```python
from build123d import *

# Parameters (mm, degrees)
F0_R     = 12.425
F0_R_2   = 11.175
F1_DEPTH = 38.1
F0_R_3   = 18.425
F2_DEPTH = 2.5
F3_SIZE  = 2
F4_R     = 1
F5_W     = 26.7045460641
F5_H     = 56.1363650486
F6_DEPTH = 1
F8_DEPTH = 50


with BuildPart() as f1:
    # F0 (on Top) → F1 (new body)
    with BuildSketch(Plane.XY):
        Circle(F0_R)
        Circle(F0_R_2, mode=Mode.SUBTRACT)
    extrude(amount=-F1_DEPTH)

    # F0 (on Top) → F2 (join)
    with BuildSketch(Plane.XY):
        Circle(F0_R_3)
        Circle(F0_R, mode=Mode.SUBTRACT)
        Circle(F0_R)
        Circle(F0_R_2, mode=Mode.SUBTRACT)
    extrude(amount=F2_DEPTH)

    # F3
    f3_edges = [f1.edges().sort_by_distance(p)[0] for p in [
        (-18.425, 0, 2.5),
    ]]
    chamfer(f3_edges, length=F3_SIZE)

    # F4
    f4_edges = [f1.edges().sort_by_distance(p)[0] for p in [
        (-11.175, 0, 2.5),
    ]]
    fillet(f4_edges, radius=F4_R)

    # F5 (on Right) → F6 (cut)
    with BuildSketch(Plane.YZ):
        with Locations((13.3522730321, -17.5000005402)):
            Rectangle(F5_W, F5_H)
    extrude(amount=-F6_DEPTH, mode=Mode.SUBTRACT)

    # F7 (on Top) → F8 (cut, symmetric)
    with BuildSketch(Plane.XY):
        Polygon((5.7434663265, -25.6659543005), (0, -11.8), (-5.7434663265, -25.6659543005), align=None)
    extrude(amount=F8_DEPTH, both=True, mode=Mode.SUBTRACT)


solid = f1.part
```
Here's how the part is built. I have some questions about the finished solid (model axes, mm). A direction names the side the tool comes from. Round coordinates to 2 decimals unless told otherwise and drop trailing zeros. Write each loop counter-clockwise with the first axis right and the second up, starting at its lowest first coordinate (ties: lowest second). Pieces come first, ordered by that corner, then holes.
Q1. Which directions (+Z, -Z, +X, -X, +Y, -Y) give clear straight access to the entire face, cutting with the end or side of a thin tool? Please do faces 1 (the flat face through (13, 0, 0)), 2 (the flat face through (-14, 0, 0)), 3 (the flat face through (-1, 12, -15)).
Q2. Please list where these lines run through material, in increasing order: probe 1 along X at (y, z) = (0, -26) (3 decimals); probe 2 along Z at (x, y) = (-11, 13.5); probe 3 along Y at (x, z) = (-2.5, -26).
Q3. Will these pins go through, and if not, where does the flat tip stop? P1, Ø12, axis at y = 1.5, z = -23, coming from the -X side (3 decimals); P2, Ø2, axis at y = 2.5, z = -29.5, coming from the -X side; P3, Ø3, axis at x = 5, z = -15.5, coming from the +Y side.
Q4. If we section it at A-A on z = -15.5: Write out the boundary of the cut face in (x, y) (3 decimals).
Answer below:
1. face 1: -Z, +X
1. face 2: -Z, -X
1. face 3: +Z, -Z, +Y
2. probe 1: x = -12.425 to -11.175, 11.175 to 12.425
2. probe 2: z = 0 to 1.51
2. probe 3: y = -12.17 to -10.89, 10.89 to 12.17
3. P1: stops at x = -12.425
3. P2: stops at x = -12.33
3. P3: stops at y = 11.92
4. outline: (-1, 11.13) - (-1, 12.385) arc R12.425 ccw to (-0.258, -12.422) - (0, -11.8) - (0.258, -12.422) arc R12.425 ccw to (0, 12.425) - (0, 11.175) arc R11.175 cw (long way) to start
